Autodesk Inventor part; units mm, degrees
ref_plane "YZ Plane" through (0, 0, 0) normal (1, 0, 0) x (0, 1, 0)
ref_plane "XZ Plane" through (0, 0, 0) normal (0, 1, 0) x (-1, 0, 0)
ref_plane "XY Plane" through (0, 0, 0) normal (0, 0, 1) x (1, 0, 0)
sketch "Sketch1" plane through (0, 0, 0) normal (0, 1, 0) x (-1, 0, 0)
  line L0 (-30, 30) -> (30, 30)
  line L1 (30, 30) -> (30, -30)
  line L2 (30, -30) -> (-30, -30)
  line L3 (-30, -30) -> (-30, 30)
  line L4 (-30, 30) -> (30, -30) construction
  line L5 (30, 30) -> (-30, -30) construction
  line L6 (-34, 34) -> (34, 34)
  line L7 (34, 34) -> (34, -34)
  line L8 (34, -34) -> (-34, -34)
  line L9 (-34, -34) -> (-34, 34)
  line L10 (-34, 34) -> (34, -34) construction
  line L11 (34, 34) -> (-34, -34) construction
  point P0 (0, 0)
  dimension "d0" = 60
  dimension "d1" = 4
  dimension "d2" = 4
extrude "Extrusion1" add sketch "Sketch1" along normal blind 90
sketch "Sketch2" plane through (34, 0, 34) normal (1, 0, 0) x (0, 0, -1)
  line L0 (31.5, 87) -> (36.5, 87)
  line L1 (36.5, 87) -> (36.5, 84)
  line L2 (36.5, 84) -> (31.5, 84)
  line L3 (31.5, 84) -> (31.5, 87)
  line L4 (31.5, 87) -> (36.5, 84) construction
  line L5 (36.5, 87) -> (31.5, 84) construction
  line L6 (0, 90) -> (68, 90)
  point P0 (34, 0)
  point P1 (34, 85.5)
  dimension "d5" = 3
  dimension "d6" = 3
  dimension "d7" = 5
extrude "Extrusion2" cut sketch "Sketch2" against normal up to surface (4 mm away)
pattern_circular "Circular Pattern1" count 4 over 360 about axis through (0, -10, 0) along (0, 1, 0) of "Extrusion2"
sketch "Sketch3" plane through (0, 0, 0) normal (0, -1, 0) x (1, 0, 0)
  arc A0 (-43.6, 0) -> (43.6, 0) centre (0, 0) ccw
  arc A1 (-46.1, 0) -> (46.1, 0) centre (0, 0) ccw
  line L0 (43.6, 0) -> (46.1, 0)
  line L1 (-46.1, 0) -> (-43.6, 0)
  line L2 (0, 0) -> (7.0498, 0) construction
  dimension "d14" = 2.5
  dimension "d17" = 43.6
revolve "Revolution1" add sketch "Sketch3" angle 180 about axis through (0, 0, 0) along (-1, 0, 0)
ref_plane "Work Plane1" through (0, -21, 0) normal (0, -1, 0) x (1, 0, 0)
properties part number "box-v1"
Verification items for the finished model (mm, model axes). A direction names the side the tool comes from. Coordinates: 2 decimals unless noted, no trailing zeros. Write each loop counter-clockwise with the first axis right and the second up, starting at its lowest first coordinate (ties: lowest second). Pieces come first, ordered by that corner, then holes. Notation, with made-up numbers: M 54,63.5 L 109,63.5 A21 ccw 109,95.5 Z; hole C 32,52 d2. An arc over 180 degrees is marked long. Answer as a JSON object with one key per item and string values. Group by question number.
(1) Cross-section at C-C, the plane x = 20.5. Record the cut outline in (y, z), and give its area (3 significant figures).
(2) Cross-section at B-B, the plane z = 14.5. Record the cut outline in (x, y), and give its area (3 significant figures).
(3) Cross-section at A-A, the plane y = 18. Record the cut outline in (x, z), and give its area (3 significant figures).
(4) Gauge pin test, flat ends, axial feed: pin 1 (1.5 mm diameter, centred on x = -31, y = 85.5, fed in from -Z); pin 2 (2 mm diameter, centred on x = -0.5, z = 31.5, fed in from -Y); pin 3 (1.5 mm diameter, centred on y = 86, z = -32.5, fed in from +X). Record the tip position at first contact, or that the pin passes through.
(5) Material ranges on line 1 (X direction, y = 15.5, z = 7); line 2 (Z direction, x = 18.5, y = -32), recorded low to high.
(6) Tool access check on faces 1 (the face through (-32, 86, 2.5)), 2 (the face through (0, 44, 30)), 3 (the face through (-2.5, 85, 32)). Record the directions out of +Z, -Z, +X, -X, +Y, -Y that give a thin tool (end or side, any length) a straight path to the whole face; none if there is none.
(7) Release check for a two-part mould opening along Y. For faces 4 (the face through (0, 87, 32)), 5 (the face through (30.4, 90, 0.2)), 6 (the face through (-33, 0, 33)), 7 (the face through (0, 44, -30)) record: +Y half, -Y half, draft (parallel to the pull), parting line (faces both ways), or undercut.
(8) Cross-section at D-D, the plane x = -36. Record the cut outline in (y, z).
Reply:
{
 "1": {"outline": "M 0,-41.29 L 0,-38.48 A38.48 cw 0,38.48 L 0,41.29 A41.29 ccw Z; M 0,-34 L 90,-34 L 90,-30 L 0,-30 Z; M 0,30 L 90,30 L 90,34 L 0,34 Z", "area": "1,070 mm²"},
 "2": {"outline": "M -43.76,0 A43.76 ccw 43.76,0 L 41.12,0 A41.12 cw -41.12,0 Z; M -34,0 L -30,0 L -30,90 L -34,90 Z; M 30,0 L 34,0 L 34,90 L 30,90 Z", "area": "1,070 mm²"},
 "3": {"outline": "M -34,-34 L 34,-34 L 34,34 L -34,34 Z; hole M -30,-30 L 30,-30 L 30,30 L -30,30 Z", "area": "1,020 mm²"},
 "4": {"pin 1": "z = -34", "pin 2": "y = -34.56", "pin 3": "x = 34"},
 "5": {"line 1": "-34 to -30, 30 to 34", "line 2": "-27.55 to -23.12, 23.12 to 27.55"},
 "6": {"face 1": "+X, -X", "face 2": "+Y", "face 3": "+Z, -Z"},
 "7": {"face 4": "undercut", "face 5": "+Y half", "face 6": "-Y half", "face 7": "draft"},
 "8": {"outline": "M 0,-28.8 L 0,-24.6 A24.6 cw 0,24.6 L 0,28.8 A28.8 ccw Z"}
}
